```python
from build123d import *

# Parameters (mm, degrees)
SKETCH_1_W          = 17
SKETCH_1_H          = 20
EXTRUDE_1_DEPTH     = 3.2
SKETCH_2_W          = 17
SKETCH_2_H          = 3.2
EXTRUDE_2_DEPTH     = 16.8
EXTRUDE_3_DEPTH     = 2.6
CUT_EXTRUDE_1_DEPTH = 22.318771072


with BuildPart() as part:
    # 草图1 → 凸台-拉伸1 (new body)
    with BuildSketch(Plane.XY):
        Rectangle(SKETCH_1_W, SKETCH_1_H)
    extrude(amount=EXTRUDE_1_DEPTH)

    # 草图2 → 凸台-拉伸2 (add)
    with BuildSketch(Plane.XY.offset(3.2)):
        with Locations((0, -8.4)):
            Rectangle(SKETCH_2_W, SKETCH_2_H)
    extrude(amount=EXTRUDE_2_DEPTH)

    # 草图3 → 凸台-拉伸3 (add)
    with BuildSketch(Plane.ZY.offset(8.5)):
        Polygon((3.2, 10), (20, -6.8), (3.2, -6.8), align=None)
    extrude_3 = extrude(amount=-EXTRUDE_3_DEPTH)

    # 镜向1: 凸台-拉伸3 across plane
    add(extrude_3.mirror(Plane(origin=(0, 0, 0), x_dir=(0, 0, 1), z_dir=(1, 0, 0))))

    # 草图4 → 切除-拉伸1 (cut, through all)
    with BuildSketch(Plane.XY.offset(3.2)):
        with BuildLine():
            Line((3, 3.495071076), (3, 0.995071076))
            ThreePointArc((3, 0.995071076), (0, -2.004928924), (-3, 0.995071076))
            Line((-3, 0.995071076), (-3, 3.495071076))
            ThreePointArc((-3, 3.495071076), (0, 6.495071076), (3, 3.495071076))
        make_face()
    cut_extrude_1 = extrude(amount=-CUT_EXTRUDE_1_DEPTH, mode=Mode.SUBTRACT)

    # 镜向2: 切除-拉伸1 across plane
    add(cut_extrude_1.mirror(Plane(origin=(0, -5, 5), x_dir=(0, 0.7071067811865479, 0.7071067811865472), z_dir=(0, -0.7071067811865474, 0.7071067811865478))), mode=Mode.SUBTRACT)


solid = part.part
```
Part model, mm, in its own coordinate system. A direction names the side the tool comes from. Round coordinates to 2 decimals unless told otherwise and drop trailing zeros. Loops run counter-clockwise (first coordinate to the right, second up) from the corner with the lowest first, then second, coordinate; pieces in that order, holes last.
1. Slice it at D-D (y = -4.5). Give the cut face in (x, z).
Solutions:
outline: (-8.5, 0) - (8.5, 0) - (8.5, 17.7) - (5.9, 17.7) - (5.9, 3.2) - (-5.9, 3.2) - (-5.9, 17.7) - (-8.5, 17.7) - close
2. Slice it at A-A (y = 3). Give the cut face in (x, z).
Solutions:
outline: (-8.5, 0) - (-3, 0) - (-3, 3.2) - (-5.9, 3.2) - (-5.9, 10.2) - (-8.5, 10.2) - close; (3, 0) - (8.5, 0) - (8.5, 10.2) - (5.9, 10.2) - (5.9, 3.2) - (3, 3.2) - close
3. Drill centre lines: line 1 along X through (y, z) = (5.75, 7.25); line 2 along Y through (x, z) = (4.5, 7); line 3 along Z through (x, y) = (-3, 7.75). Where is each one in solid material? Low to high.
Solutions:
line 1: x = -8.5 to -5.9, 5.9 to 8.5
line 2: y = -10 to -6.8
line 3: z = 0 to 3.2
4. 3-axis set-ups, long thin cutter, end or side, ignore diameter. For faces 4 (the face through (-3, -6.8, 10)), 5 (the face through (-0.066, -8.378, 16.494)), 6 (the face through (3, 2, 2)): which of +Z, -Z, +X, -X, +Y, -Y reach the whole face in a straight line?
Solutions:
face 4: +Z, +Y
face 5: +Y, -Y
face 6: +Z, -Z
5. Slice it at C-C (x = 7). Give the cut face in (y, z).
Solutions:
outline: (-10, 0) - (10, 0) - (10, 3.2) - (-6.8, 20) - (-10, 20) - close
6. Two-plate mould, pull along X, no slides. Class faces 1 (the face through (0, -8, 20)), 2 (the face through (8.5, -2, 8)), 3 (the face through (0.066, -8.378, 7.996)): pulls with the +X half, pulls with the -X half, needs draft (parallel to the pull), parting line crosses it, or undercut.
Solutions:
face 1: needs draft
face 2: pulls with the +X half
face 3: undercut
7. Slice it at B-B (x = 0). Give the cut face in (y, z), and give its area (3 significant figures).
Solutions:
outline: (-10, 0) - (-2, 0) - (-2, 3.2) - (-6.8, 3.2) - (-6.8, 8) - (-10, 8) - close; (-10, 16.5) - (-6.8, 16.5) - (-6.8, 20) - (-10, 20) - close; (6.5, 0) - (10, 0) - (10, 3.2) - (6.5, 3.2) - close
area: 63.4 mm2
8. Flat gauge pins, fed straight in: pin 1 (1 mm diameter, centred on x = -5.5, z = 16, fed in from +Y); pin 2 (9.5 mm diameter, centred on x = -2, z = 8.5, fed in from +Y); pin 3 (5 mm diameter, centred on x = 0.5, y = 0, fed in from +Z). Where does each tip first touch, or does it go through?
Solutions:
pin 1: stops at y = -2.5
pin 2: stops at y = 7.41
pin 3: stops at z = 3.2
